from build123d import *

# Parameters (mm, degrees)
SKETCH1_W            = 260
SKETCH1_H            = 440
EXTRUDE1_DEPTH       = 10
SKETCH3_W            = 260
SKETCH3_H            = 40
EXTRUDE3_DEPTH       = 10
SKETCH4_W            = 20
SKETCH4_H            = 10
CUT_EXTRUDE1_DEPTH   = 10
EXTRUDE4_DEPTH       = 10
MIRROR2_COPY_1_DEPTH = 10
MIRROR3_COPY_1_DEPTH = 10
MIRROR3_COPY_2_DEPTH = 10
MIRROR3_COPY_3_DEPTH = 10
MIRROR4_COPY_1_DEPTH = 10
MIRROR4_COPY_2_DEPTH = 10
MIRROR4_COPY_3_DEPTH = 10
M4_CLEARANCE_HOLE1_D = 4.5
SKETCH8_W            = 20
SKETCH8_H            = 10
CUT_EXTRUDE2_DEPTH   = 10
EXTRUDE5_DEPTH       = 10
CHAMFER1_SIZE        = 10
SKETCH10_W           = 170
SKETCH10_H           = 20
EXTRUDE6_DEPTH       = 10
CHAMFER2_SIZE        = 5


with BuildPart() as part:
    # Sketch1 → Extrude1 (new body)
    with BuildSketch(Plane(origin=(0, 0, 0), x_dir=(1, 0, 0), z_dir=(0, 1, 0))):
        Rectangle(SKETCH1_W, SKETCH1_H)
    extrude(amount=EXTRUDE1_DEPTH)

    # Sketch3 → Extrude3 (add)
    with BuildSketch(Plane(origin=(0, 10, 0), x_dir=(1, 0, 0), z_dir=(0, 1, 0))):
        with Locations((0, 240)):
            Rectangle(SKETCH3_W, SKETCH3_H)
    extrude(amount=-EXTRUDE3_DEPTH)

    # Sketch4 → Cut-Extrude1 (cut)
    with BuildSketch(Plane(origin=(130, 0, -206), x_dir=(1, 0, 0), z_dir=(0, -1, 0))):
        with Locations((-235, 391)):
            Rectangle(SKETCH4_W, SKETCH4_H)
        with Locations((-195, 391)):
            Rectangle(SKETCH4_W, SKETCH4_H)
        with Locations((-65, 391)):
            Rectangle(SKETCH4_W, SKETCH4_H)
        with Locations((-25, 391)):
            Rectangle(SKETCH4_W, SKETCH4_H)
        with Locations((-235, 175)):
            Rectangle(SKETCH4_W, SKETCH4_H)
        with Locations((-195, 175)):
            Rectangle(SKETCH4_W, SKETCH4_H)
        with Locations((-65, 175)):
            Rectangle(SKETCH4_W, SKETCH4_H)
        with Locations((-25, 175)):
            Rectangle(SKETCH4_W, SKETCH4_H)
        with Locations((-235, -15)):
            Rectangle(SKETCH4_W, SKETCH4_H)
        with Locations((-195, -15)):
            Rectangle(SKETCH4_W, SKETCH4_H)
        with Locations((-65, -15)):
            Rectangle(SKETCH4_W, SKETCH4_H)
        with Locations((-25, -15)):
            Rectangle(SKETCH4_W, SKETCH4_H)
    extrude(amount=-CUT_EXTRUDE1_DEPTH, mode=Mode.SUBTRACT)

    # Sketch5 → Extrude4 (cut)
    with BuildSketch(Plane(origin=(0, 0, 0), x_dir=(-1, 0, 0), z_dir=(0, -1, 0))):
        with BuildLine():
            Line((96.5, -190), (95, -190))
            Line((95, -190), (95, -188.5))
            ThreePointArc((95, -188.5), (93.939339828, -191.060660172), (96.5, -190))
        make_face()
        with BuildLine():
            Line((115, -190), (113.5, -190))
            ThreePointArc((113.5, -190), (116.060660172, -191.060660172), (115, -188.5))
            Line((115, -188.5), (115, -190))
        make_face()
        with BuildLine():
            Line((115, -180), (113.5, -180))
            ThreePointArc((113.5, -180), (116.060660172, -178.939339828), (115, -181.5))
            Line((115, -181.5), (115, -180))
        make_face()
        with BuildLine():
            Line((96.5, -180), (95, -180))
            Line((95, -180), (95, -181.5))
            ThreePointArc((95, -181.5), (93.939339828, -178.939339828), (96.5, -180))
        make_face()
    extrude4 = extrude(amount=-EXTRUDE4_DEPTH, mode=Mode.SUBTRACT)

    # Mirror1: Extrude4 across plane
    add(extrude4.mirror(Plane(origin=(-85, 0, 0), x_dir=(0, 0, 1), z_dir=(1, 0, 0))), mode=Mode.SUBTRACT)

    # Mirror2: Extrude4 across plane
    add(extrude4.mirror(Plane(origin=(0, 0, 0), x_dir=(0, 0, 1), z_dir=(1, 0, 0))), mode=Mode.SUBTRACT)

    # Mirror2 copy 1 sketch → Mirror2 copy 1 (cut)
    with BuildSketch(Plane(origin=(170, 0, 0), x_dir=(-1, 0, 0), z_dir=(0, -1, 0))):
        with BuildLine():
            Line((96.5, -190), (95, -190))
            Line((95, -190), (95, -188.5))
            ThreePointArc((95, -188.5), (93.939339828, -191.060660172), (96.5, -190))
        make_face()
        with BuildLine():
            Line((115, -190), (113.5, -190))
            ThreePointArc((113.5, -190), (116.060660172, -191.060660172), (115, -188.5))
            Line((115, -188.5), (115, -190))
        make_face()
        with BuildLine():
            Line((115, -180), (113.5, -180))
            ThreePointArc((113.5, -180), (116.060660172, -178.939339828), (115, -181.5))
            Line((115, -181.5), (115, -180))
        make_face()
        with BuildLine():
            Line((96.5, -180), (95, -180))
            Line((95, -180), (95, -181.5))
            ThreePointArc((95, -181.5), (93.939339828, -178.939339828), (96.5, -180))
        make_face()
    extrude(amount=-MIRROR2_COPY_1_DEPTH, mode=Mode.SUBTRACT)

    # Mirror3: Extrude4 across plane
    add(extrude4.mirror(Plane(origin=(0, 0, 77), x_dir=(1, 0, 0), z_dir=(0, 0, -1))), mode=Mode.SUBTRACT)

    # Mirror3 copy 1 sketch → Mirror3 copy 1 (cut)
    with BuildSketch(Plane(origin=(-170, 0, 154), x_dir=(1, 0, 0), z_dir=(0, -1, 0))):
        with BuildLine():
            Line((96.5, -190), (95, -190))
            Line((95, -190), (95, -188.5))
            ThreePointArc((95, -188.5), (93.939339828, -191.060660172), (96.5, -190))
        make_face()
        with BuildLine():
            Line((115, -190), (113.5, -190))
            ThreePointArc((113.5, -190), (116.060660172, -191.060660172), (115, -188.5))
            Line((115, -188.5), (115, -190))
        make_face()
        with BuildLine():
            Line((115, -180), (113.5, -180))
            ThreePointArc((113.5, -180), (116.060660172, -178.939339828), (115, -181.5))
            Line((115, -181.5), (115, -180))
        make_face()
        with BuildLine():
            Line((96.5, -180), (95, -180))
            Line((95, -180), (95, -181.5))
            ThreePointArc((95, -181.5), (93.939339828, -178.939339828), (96.5, -180))
        make_face()
    extrude(amount=-MIRROR3_COPY_1_DEPTH, mode=Mode.SUBTRACT)

    # Mirror3 copy 2 sketch → Mirror3 copy 2 (cut)
    with BuildSketch(Plane(origin=(0, 0, 154), x_dir=(1, 0, 0), z_dir=(0, -1, 0))):
        with BuildLine():
            Line((96.5, -190), (95, -190))
            Line((95, -190), (95, -188.5))
            ThreePointArc((95, -188.5), (93.939339828, -191.060660172), (96.5, -190))
        make_face()
        with BuildLine():
            Line((115, -190), (113.5, -190))
            ThreePointArc((113.5, -190), (116.060660172, -191.060660172), (115, -188.5))
            Line((115, -188.5), (115, -190))
        make_face()
        with BuildLine():
            Line((115, -180), (113.5, -180))
            ThreePointArc((113.5, -180), (116.060660172, -178.939339828), (115, -181.5))
            Line((115, -181.5), (115, -180))
        make_face()
        with BuildLine():
            Line((96.5, -180), (95, -180))
            Line((95, -180), (95, -181.5))
            ThreePointArc((95, -181.5), (93.939339828, -178.939339828), (96.5, -180))
        make_face()
    extrude(amount=-MIRROR3_COPY_2_DEPTH, mode=Mode.SUBTRACT)

    # Mirror3 copy 3 sketch → Mirror3 copy 3 (cut)
    with BuildSketch(Plane(origin=(170, 0, 154), x_dir=(-1, 0, 0), z_dir=(0, -1, 0))):
        with BuildLine():
            Line((96.5, 190), (95, 190))
            Line((95, 190), (95, 188.5))
            ThreePointArc((95, 188.5), (93.939339828, 191.060660172), (96.5, 190))
        make_face()
        with BuildLine():
            Line((115, 190), (113.5, 190))
            ThreePointArc((113.5, 190), (116.060660172, 191.060660172), (115, 188.5))
            Line((115, 188.5), (115, 190))
        make_face()
        with BuildLine():
            Line((115, 180), (113.5, 180))
            ThreePointArc((113.5, 180), (116.060660172, 178.939339828), (115, 181.5))
            Line((115, 181.5), (115, 180))
        make_face()
        with BuildLine():
            Line((96.5, 180), (95, 180))
            Line((95, 180), (95, 181.5))
            ThreePointArc((95, 181.5), (93.939339828, 178.939339828), (96.5, 180))
        make_face()
    extrude(amount=-MIRROR3_COPY_3_DEPTH, mode=Mode.SUBTRACT)

    # Mirror4: Extrude4 across plane
    add(extrude4.mirror(Plane.XY.offset(-18)), mode=Mode.SUBTRACT)

    # Mirror4 copy 1 sketch → Mirror4 copy 1 (cut)
    with BuildSketch(Plane(origin=(-170, 0, -36), x_dir=(1, 0, 0), z_dir=(0, -1, 0))):
        with BuildLine():
            Line((96.5, -190), (95, -190))
            Line((95, -190), (95, -188.5))
            ThreePointArc((95, -188.5), (93.939339828, -191.060660172), (96.5, -190))
        make_face()
        with BuildLine():
            Line((115, -190), (113.5, -190))
            ThreePointArc((113.5, -190), (116.060660172, -191.060660172), (115, -188.5))
            Line((115, -188.5), (115, -190))
        make_face()
        with BuildLine():
            Line((115, -180), (113.5, -180))
            ThreePointArc((113.5, -180), (116.060660172, -178.939339828), (115, -181.5))
            Line((115, -181.5), (115, -180))
        make_face()
        with BuildLine():
            Line((96.5, -180), (95, -180))
            Line((95, -180), (95, -181.5))
            ThreePointArc((95, -181.5), (93.939339828, -178.939339828), (96.5, -180))
        make_face()
    extrude(amount=-MIRROR4_COPY_1_DEPTH, mode=Mode.SUBTRACT)

    # Mirror4 copy 2 sketch → Mirror4 copy 2 (cut)
    with BuildSketch(Plane(origin=(0, 0, -36), x_dir=(1, 0, 0), z_dir=(0, -1, 0))):
        with BuildLine():
            Line((96.5, -190), (95, -190))
            Line((95, -190), (95, -188.5))
            ThreePointArc((95, -188.5), (93.939339828, -191.060660172), (96.5, -190))
        make_face()
        with BuildLine():
            Line((115, -190), (113.5, -190))
            ThreePointArc((113.5, -190), (116.060660172, -191.060660172), (115, -188.5))
            Line((115, -188.5), (115, -190))
        make_face()
        with BuildLine():
            Line((115, -180), (113.5, -180))
            ThreePointArc((113.5, -180), (116.060660172, -178.939339828), (115, -181.5))
            Line((115, -181.5), (115, -180))
        make_face()
        with BuildLine():
            Line((96.5, -180), (95, -180))
            Line((95, -180), (95, -181.5))
            ThreePointArc((95, -181.5), (93.939339828, -178.939339828), (96.5, -180))
        make_face()
    extrude(amount=-MIRROR4_COPY_2_DEPTH, mode=Mode.SUBTRACT)

    # Mirror4 copy 3 sketch → Mirror4 copy 3 (cut)
    with BuildSketch(Plane(origin=(170, 0, -36), x_dir=(-1, 0, 0), z_dir=(0, -1, 0))):
        with BuildLine():
            Line((96.5, 190), (95, 190))
            Line((95, 190), (95, 188.5))
            ThreePointArc((95, 188.5), (93.939339828, 191.060660172), (96.5, 190))
        make_face()
        with BuildLine():
            Line((115, 190), (113.5, 190))
            ThreePointArc((113.5, 190), (116.060660172, 191.060660172), (115, 188.5))
            Line((115, 188.5), (115, 190))
        make_face()
        with BuildLine():
            Line((115, 180), (113.5, 180))
            ThreePointArc((113.5, 180), (116.060660172, 178.939339828), (115, 181.5))
            Line((115, 181.5), (115, 180))
        make_face()
        with BuildLine():
            Line((96.5, 180), (95, 180))
            Line((95, 180), (95, 181.5))
            ThreePointArc((95, 181.5), (93.939339828, 178.939339828), (96.5, 180))
        make_face()
    extrude(amount=-MIRROR4_COPY_3_DEPTH, mode=Mode.SUBTRACT)

    # M4 Clearance Hole1 (through all)
    with Locations(Plane(origin=(0, 10, 0), x_dir=(1, 0, 0), z_dir=(0, 1, 0))):
        with Locations((-85, 221), (85, 221), (85, 31), (-85, 31), (-85, -185), (85, -185)):
            Hole(M4_CLEARANCE_HOLE1_D / 2)

    # Sketch8 → Cut-Extrude2 (cut)
    with BuildSketch(Plane(origin=(130, 0, -206), x_dir=(1, 0, 0), z_dir=(0, -1, 0))):
        with Locations((-130, 165)):
            Rectangle(SKETCH8_W, SKETCH8_H)
        with Locations((-130, -5)):
            Rectangle(SKETCH8_W, SKETCH8_H)
    extrude(amount=-CUT_EXTRUDE2_DEPTH, mode=Mode.SUBTRACT)

    # Sketch9 → Extrude5 (cut)
    with BuildSketch(Plane.XZ):
        with BuildLine():
            Line((-10, -44.5), (-10, -46))
            Line((-10, -46), (-8.5, -46))
            ThreePointArc((-8.5, -46), (-11.060660172, -47.060660172), (-10, -44.5))
        make_face()
        with BuildLine():
            Line((-10, -36), (-8.5, -36))
            ThreePointArc((-8.5, -36), (-11.060660172, -34.939339828), (-10, -37.5))
            Line((-10, -37.5), (-10, -36))
        make_face()
        with BuildLine():
            Line((10, -36), (10, -37.5))
            ThreePointArc((10, -37.5), (11.060660172, -34.939339828), (8.5, -36))
            Line((8.5, -36), (10, -36))
        make_face()
        with BuildLine():
            Line((8.5, -46), (10, -46))
            Line((10, -46), (10, -44.5))
            ThreePointArc((10, -44.5), (11.060660172, -47.060660172), (8.5, -46))
        make_face()
    extrude5 = extrude(amount=-EXTRUDE5_DEPTH, mode=Mode.SUBTRACT)

    # Mirror5: Extrude5 across plane
    add(extrude5.mirror(Plane.XY.offset(-126)), mode=Mode.SUBTRACT)

    # Chamfer1
    chamfer1_edges = [part.edges().sort_by_distance(p)[0] for p in [
        (130, 5, 220),
        (-130, 5, 220),
    ]]
    chamfer(chamfer1_edges, length=CHAMFER1_SIZE)

    # Sketch10 → Extrude6 (cut)
    with BuildSketch(Plane(origin=(0, 10, 0), x_dir=(1, 0, 0), z_dir=(0, 1, 0))):
        with Locations((0, 250)):
            Rectangle(SKETCH10_W, SKETCH10_H)
    extrude(amount=-EXTRUDE6_DEPTH, mode=Mode.SUBTRACT)

    # Chamfer2
    chamfer2_edges = [part.edges().sort_by_distance(p)[0] for p in [
        (-130, 5, -260),
        (130, 5, -260),
        (-85, 5, -240),
        (-85, 5, -260),
        (85, 5, -260),
        (85, 5, -240),
    ]]
    chamfer(chamfer2_edges, length=CHAMFER2_SIZE)


solid = part.part
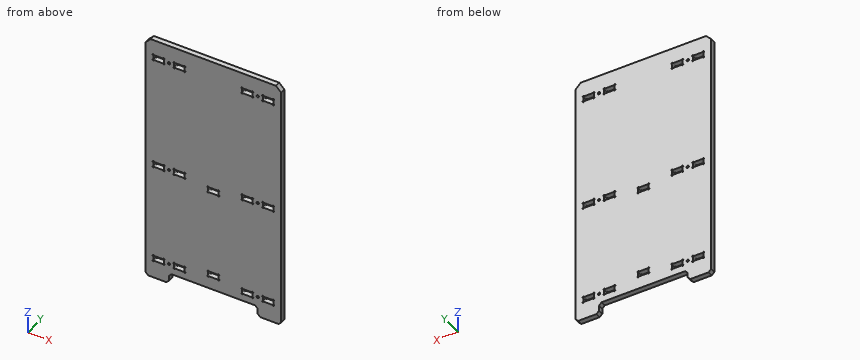
Input: part model. Units: mm. Frame: model coordinates. Coordinates: 2 decimals unless noted, no trailing zeros. Order: outer loops, then holes, each group sorted by start corner. A loop starts at its lowest first (then second) coordinate and runs counter-clockwise, first axis right, second up. Notation, with made-up numbers: M 53.25,-33.5 L 87.25,-33.5 A7 cw 87.25,-20.5 Z; hole C 89.5,84 d7. An arc over 180 degrees is marked long. Write item = value, one per line. Start each with the question number.
(1) Line query: line 1 along Z through (x, y) = (-99, 7.5); line 2 along Z through (x, y) = (-58.5, 9.25); line 3 along Z through (x, y) = (-13, 0.75). Output: solid intervals per line, ascending. Write a range as [from, to].
(2) Section B-B on y = 2.5. Give the number of separate pieces and of enclosed holes in the cut face, and give its area (3 significant figures).
(3) Section A-A on x = 61. Output: boundary loops of the cut face in (y, z).
(4) First-contact query: P1, Ø5, axis at x = 82, y = 7, coming from the -Z side; P2, Ø1, axis at x = 47, y = 3, coming from the -Z side. Flat tips, straight axial feed; report the tip coordinate or a pass-through.
Result set:
q1.line_1 = [-260, -226], [-216, -36], [-26, 180], [190, 220]
q1.line_2 = [-240, -226], [-216, -36], [-26, 180], [190, 220]
q1.line_3 = [-240, 220]
q2.separate_pieces = 1
q2.enclosed_holes = 20
q2.area = 118,000 mm²
q3.outline = M 0,-240 L 10,-240 L 10,-226 L 0,-226 Z; M 0,-216 L 10,-216 L 10,-36 L 0,-36 Z; M 0,-26 L 10,-26 L 10,180 L 0,180 Z; M 0,190 L 10,190 L 10,220 L 0,220 Z
q4.P1 = -244.5
q4.P2 = -240
